The figure shows three views and two pictorial views of one solid part (mm, origin at its lowest corner). Answer the questions. A direction names the side the tool comes from. Round coordinates to 2 decimals unless told otherwise and drop trailing zeros. Order: outer loops, then holes, each group sorted by start corner. A loop starts at its lowest first (then second) coordinate and runs counter-clockwise, first axis right, second up. Notation, with made-up numbers: (33, 12.25) -> (47, 12.25) arc R13 cw to (47, 36.25) -> close; hole circle Ø9 at (79, 47.5). An arc over 180 degrees is marked (long way). Return JSON: item names as keys, results as strings. Group by question number.
(1) Determine the mould class of the marked faces 6, 7 and 8 for opening direction X: +X half, -X half, draft (parallel to the pull), parting line (faces both ways), or undercut.
(2) The part is cut by section B-B (y = 29). Determine the outline of the cut face in (x, z).
(3) The part is cut by section D-D (y = 60.5). Determine the outline of the cut face in (x, z).
(4) The part is cut by section C-C (z = 16). Determine the outline of the cut face in (x, y).
(5) The part is cut by section A-A (x = 28.5). Determine the outline of the cut face in (y, z).
(6) Which of the six approach directions +Z, -Z, +X, -X, +Y, -Y give full straight-line access (tool end or side, diameter ignored) to the marked faces 1, 2, 3, 4 and 5?
(7) Each of these flat-tipped pins is pushed along its axis until it touches: pin 1 (1 mm diameter, centred on y = 35.5, z = 59, fed in from -X); pin 2 (8 mm diameter, centred on x = 4, z = 7, fed in from -Y); pin 3 (8 mm diameter, centred on x = 3.5, y = 37, fed in from -Z); pin 4 (3 mm diameter, centred on x = 85, y = 48, fed in from +Z). Where does it stop, or does it pass through?
(8) Consider line 1 (X direction, y = 40.5, z = 16); line 2 (Y direction, x = 29.5, z = 21); line 3 (Z direction, x = 90, y = 38.5). Determine where each line is inside the solid, lowest interval first. Write a range as [from, to].
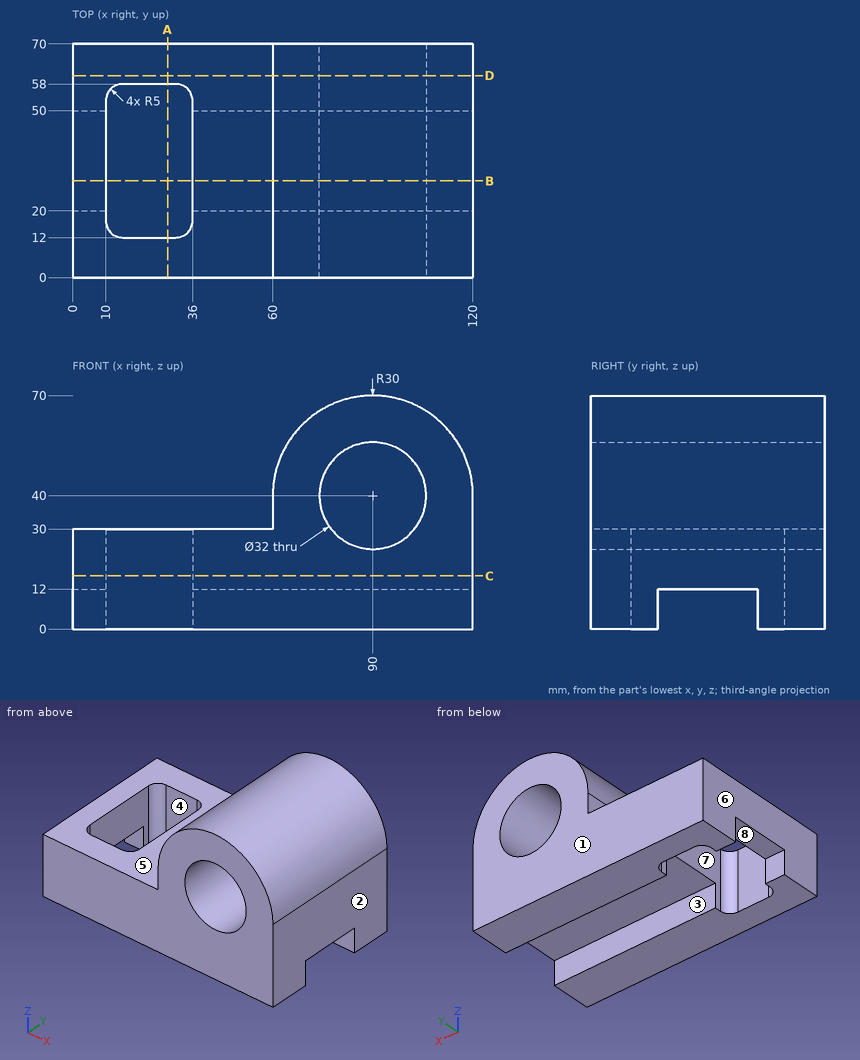
Answer below:
{
 "1": {"face 6": "-X half", "face 7": "undercut", "face 8": "draft"},
 "2": {"outline": "(0, 12) -> (10, 12) -> (10, 30) -> (0, 30) -> close; (36, 12) -> (120, 12) -> (120, 40) arc R30 ccw to (60, 40) -> (60, 30) -> (36, 30) -> close; hole circle Ø32 at (90, 40)"},
 "3": {"outline": "(0, 0) -> (120, 0) -> (120, 40) arc R30 ccw to (60, 40) -> (60, 30) -> (0, 30) -> close; hole circle Ø32 at (90, 40)"},
 "4": {"outline": "(0, 0) -> (120, 0) -> (120, 70) -> (0, 70) -> close; hole (10, 17) arc R5 ccw to (15, 12) -> (31, 12) arc R5 ccw to (36, 17) -> (36, 53) arc R5 ccw to (31, 58) -> (15, 58) arc R5 ccw to (10, 53) -> close"},
 "5": {"outline": "(0, 0) -> (12, 0) -> (12, 30) -> (0, 30) -> close; (58, 0) -> (70, 0) -> (70, 30) -> (58, 30) -> close"},
 "6": {"face 1": "+Z, -Z, +X, -X, +Y", "face 2": "+Z, -Z, +X, +Y, -Y", "face 3": "-Z, +X, -X", "face 4": "+Z, -Z", "face 5": "+Z, -X, +Y, -Y"},
 "7": {"pin 1": "stops at x = 66.38", "pin 2": "stops at y = 0", "pin 3": "stops at z = 12", "pin 4": "stops at z = 69.8"},
 "8": {"line 1": "x = [0, 10], [36, 120]", "line 2": "y = [0, 12], [58, 70]", "line 3": "z = [12, 24], [56, 70]"}
}
